Geometry check sheet. Reference: the model listing, model coordinates, mm. Coordinates: 2 decimals unless noted, no trailing zeros. Loops run counter-clockwise (first coordinate to the right, second up) from the corner with the lowest first, then second, coordinate; pieces in that order, holes last.
from build123d import *

# Parameters (mm, degrees)
SKETCH_1_R          = 102
SKETCH_1_R_2        = 87.5
SKETCH_1_R_3        = 2.6
EXTRUDE_1_DEPTH     = 5.3
SKETCH_2_R          = 3.65
SKETCH_2_R_2        = 3.15
SKETCH_2_R_3        = 4
CUT_EXTRUDE_1_DEPTH = 145.347116355


with BuildPart() as part:
    # 草图1 → 凸台-拉伸1 (new body)
    with BuildSketch(Plane(origin=(0, 0, 0), x_dir=(1, 0, 0), z_dir=(0, 1, 0))):
        with Locations(Location((0, 0, 0), (0, 0, 270))):
            Circle(SKETCH_1_R)
        with Locations(Location((0, 0, 0), (0, 0, 270))):
            Circle(SKETCH_1_R_2, mode=Mode.SUBTRACT)
        with Locations(Location((0, 94.385, 0), (0, 0, 270))):
            Circle(SKETCH_1_R_3, mode=Mode.SUBTRACT)
        with Locations(Location((94.385, 0, 0), (0, 0, 270))):
            Circle(SKETCH_1_R_3, mode=Mode.SUBTRACT)
        with Locations(Location((0, -94.385, 0), (0, 0, 270))):
            Circle(SKETCH_1_R_3, mode=Mode.SUBTRACT)
        with Locations(Location((-94.385, 0, 0), (0, 0, 270))):
            Circle(SKETCH_1_R_3, mode=Mode.SUBTRACT)
    extrude(amount=EXTRUDE_1_DEPTH)

    # 草图2 → 切除-拉伸1 (cut, through all)
    with BuildSketch(Plane.XZ):
        with Locations((70.154572481, -56.436700926)):
            Circle(SKETCH_2_R)
        with Locations((-79.620223562, 33.516861428)):
            Circle(SKETCH_2_R_2)
        with Locations((38.336469882, -75.530286573)):
            Circle(SKETCH_2_R_3)
    extrude(amount=-CUT_EXTRUDE_1_DEPTH, mode=Mode.SUBTRACT)


solid = part.part
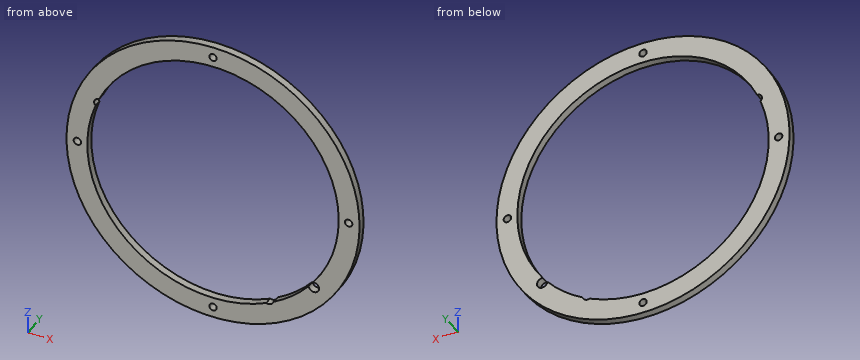
(1) Sectioned sample at D-D on z = -47. Record the cut outline in (x, y), and give its area (3 significant figures).
Findings:
outline: (-90.53, 0) - (-73.81, 0) - (-73.81, 5.3) - (-90.53, 5.3) - close; (73.81, 0) - (90.53, 0) - (90.53, 5.3) - (73.81, 5.3) - close
area: 177 mm2
(2) Sectioned sample at A-A on x = 0. Record the cut outline in (y, z) (3 decimals).
Findings:
outline: (0, -102) - (5.3, -102) - (5.3, -96.985) - (0, -96.985) - close; (0, -91.785) - (5.3, -91.785) - (5.3, -87.5) - (0, -87.5) - close; (0, 87.5) - (5.3, 87.5) - (5.3, 91.785) - (0, 91.785) - close; (0, 96.985) - (5.3, 96.985) - (5.3, 102) - (0, 102) - close
(3) Sectioned sample at B-B on z = 0. Record the cut outline in (x, y) (3 decimals).
Findings:
outline: (-102, 0) - (-96.985, 0) - (-96.985, 5.3) - (-102, 5.3) - close; (-91.785, 0) - (-87.5, 0) - (-87.5, 5.3) - (-91.785, 5.3) - close; (87.5, 0) - (91.785, 0) - (91.785, 5.3) - (87.5, 5.3) - close; (96.985, 0) - (102, 0) - (102, 5.3) - (96.985, 5.3) - close
(4) Scan lines: L1, parallel to X at y = 3.05, z = 0 (3 decimals); L2, parallel to Z at x = 70.5, y = 2.4; L3, parallel to X at y = 1.35, z = 92. Record each from-to range of solid material in increasing order.
Findings:
L1: x = -102 to -96.985, -91.785 to -87.5, 87.5 to 91.785, 96.985 to 102
L2: z = -73.71 to -60.07, -52.8 to -51.83, 51.83 to 73.71
L3: x = -44.05 to -1.04, 1.04 to 44.05
(5) Gauge pin test, flat ends, axial feed: pin 1 Ø1 at (y, z) = (2.5, -57.5) entering from +X; pin 2 Ø6 at (x, z) = (-94.385, 0) entering from -Y; pin 3 Ø1.5 at (x, y) = (-45.5, 3) entering from +Z; pin 4 Ø1.5 at (x, y) = (-9, 4) entering from +Z. Record the tip position at first contact, or that the pin passes through.
Findings:
pin 1: stops at x = 84.59
pin 2: stops at y = 0
pin 3: stops at z = 91.66
pin 4: stops at z = 101.67
(6) Sectioned sample at C-C on x = -36. Record the cut outline in (y, z), and give its area (3 significant figures).
Findings:
outline: (0, -95.44) - (5.3, -95.44) - (5.3, -79.75) - (0, -79.75) - close; (0, 79.75) - (5.3, 79.75) - (5.3, 95.44) - (0, 95.44) - close
area: 166 mm2
